For this review, use the dimensioned drawing (mm, ordinates from the lowest corner) and the shaded views. Coordinates: 2 decimals unless noted, no trailing zeros. Order: outer loops, then holes, each group sorted by start corner. A loop starts at its lowest first (then second) coordinate and runs counter-clockwise, first axis right, second up. Notation, with made-up numbers: (55, -4) -> (90, -4) arc R19 ccw to (90, 1) -> close; hole circle Ø9 at (85.25, 85.25). An arc over 180 degrees is marked (long way). Use one line per item in the form item = value. Start each with the question number.
(1) Take a section at C-C (x = 16.5). State the section outline as (y, z) points.
(2) Take a section at D-D (y = 111). State the section outline as (x, z) points.
(3) Wall thickness on line 1 along X through (y, z) = (67, 2.25); line 2 along X through (y, z) = (6.5, 0.85); line 3 along X through (y, z) = (73, 1.25): over which ranges is each line inside the solid? List them lowest first.
(4) Take a section at A-A (y = 33). State the section outline as (x, z) points.
(5) Take a section at B-B (z = 2). State the section outline as (x, y) points.
(6) Insertion check: pin 1 Ø0.9 at (y, z) = (22, 1.5) entering from -X; pin 2 Ø0.9 at (y, z) = (66.5, 2) entering from +X; pin 3 Ø0.9 at (x, z) = (1.5, 1) entering from -Y. Each pin has a flat end and moves straight along its axis. Give the tip position at first contact, or say it passes through.
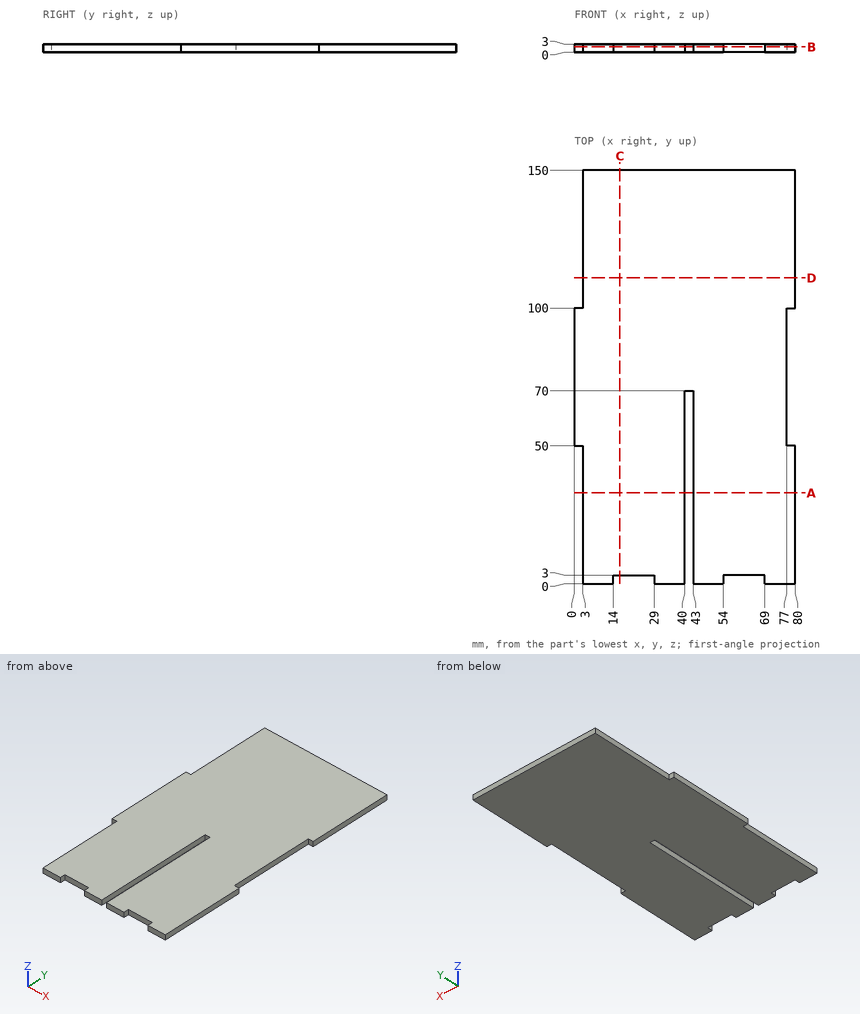
Findings:
q1.outline = (3, 0) -> (150, 0) -> (150, 3) -> (3, 3) -> close
q2.outline = (3, 0) -> (80, 0) -> (80, 3) -> (3, 3) -> close
q3.line_1 = 0 to 40, 43 to 77
q3.line_2 = 3 to 40, 43 to 80
q3.line_3 = 0 to 77
q4.outline = (3, 0) -> (40, 0) -> (40, 3) -> (3, 3) -> close; (43, 0) -> (80, 0) -> (80, 3) -> (43, 3) -> close
q5.outline = (0, 50) -> (3, 50) -> (3, 0) -> (14, 0) -> (14, 3) -> (29, 3) -> (29, 0) -> (40, 0) -> (40, 70) -> (43, 70) -> (43, 0) -> (54, 0) -> (54, 3) -> (69, 3) -> (69, 0) -> (80, 0) -> (80, 50) -> (77, 50) -> (77, 100) -> (80, 100) -> (80, 150) -> (3, 150) -> (3, 100) -> (0, 100) -> close
q6.pin_1 = 3
q6.pin_2 = 77
q6.pin_3 = 50
